Can you work these out from the model? Positions are in its coordinate system, mm. A direction names the side the tool comes from. Round coordinates to 2 decimals unless told otherwise and drop trailing zeros. Write each loop counter-clockwise with the first axis right and the second up, starting at its lowest first coordinate (ties: lowest second). Pieces come first, ordered by that corner, then holes. Notation, with made-up numbers: M 40.5,84.5 L 61.5,84.5 A4 ccw 61.5,90.5 Z; hole C 66.5,51.5 d9. An arc over 180 degrees is marked long. Answer as a JSON object with one key per item and string values. Group by question number.
1) If we mould it in two halves opening along Z, with no side actions, what happens to faces 4 (the flat face through (-35.2, 1, 13)), 5 (the flat face through (41.2, 1, -19)), 6 (the flat face through (39, 1, -12)), 7 (the flat face through (0, 1, 25))? For each: +Z half, -Z half, draft (parallel to the pull), parting line (faces both ways), or undercut.
2) Suppose I cut it at D-D, the plane y = 0.65. State how many separate pieces and enclosed holes the cut face has, and give its area (3 significant figures).
3) Suppose I cut it at B-B, the plane x = 30. Write out the boundary of the cut face in (y, z).
4) Suppose I cut it at A-A, the plane x = 19. Write out the boundary of the cut face in (y, z).
5) On a 3-axis mill with a long thin cutter (end or side, diameter ignored), from which of +Z, -Z, +X, -X, +Y, -Y can I reach the whole of each face in a straight line? I mean faces 1 (the flat face through (-40.2, 1, -19)), 2 (the flat face through (36.2, 1, -13)), 3 (the flat face through (31.2, 1, 16)). Say none if no direction works.
6) Suppose I cut it at C-C, the plane z = 0.05. Write out the boundary of the cut face in (x, y).
7) I'm going to push a flat-ended pin straight in: pin 1 Ø1 at (y, z) = (0.5, -13) entering from -X. Where does the tip first touch, or does it pass through?
8) Please list where these lines run through material, in increasing order: L1, parallel to Z at x = 30, y = 0.5; L2, parallel to X at y = 0.6, z = -17.5; L3, parallel to X at y = 0.65, z = -13.5. Write a range as [from, to].
from build123d import *

# Parameters (mm, degrees)
SKETCH2_W           = 100
SKETCH2_H           = 50
BOSS_EXTRUDE1_DEPTH = 2
SKETCH12_W          = 9.8
SKETCH12_H          = 50
SKETCH12_W_2        = 8.8
CUT_EXTRUDE8_DEPTH  = 6
SKETCH13_W          = 2
SKETCH13_H          = 7
SKETCH13_W_2        = 5
SKETCH13_H_2        = 2
CUT_EXTRUDE10_DEPTH = 6
SKETCH14_R          = 2
CUT_EXTRUDE11_DEPTH = 2


with BuildPart() as part:
    # Sketch2 → Boss-Extrude1 (new body)
    with BuildSketch(Plane(origin=(0, 0, 0), x_dir=(1, 0, 0), z_dir=(0, 1, 0))):
        Rectangle(SKETCH2_W, SKETCH2_H)
    extrude(amount=BOSS_EXTRUDE1_DEPTH)

    # Sketch12 → Cut-Extrude8 (cut)
    with BuildSketch(Plane(origin=(0, 2, 0), x_dir=(1, 0, 0), z_dir=(0, 1, 0))):
        with Locations((-45.1, 0)):
            Rectangle(SKETCH12_W, SKETCH12_H)
        with Locations((45.6, 0)):
            Rectangle(SKETCH12_W_2, SKETCH12_H)
    extrude(amount=-CUT_EXTRUDE8_DEPTH, mode=Mode.SUBTRACT)

    # Sketch13 → Cut-Extrude10 (cut)
    with BuildSketch(Plane(origin=(0, 2, 0), x_dir=(1, 0, 0), z_dir=(0, 1, 0))):
        with Locations((-29.2, 15.5)):
            Rectangle(SKETCH13_W, SKETCH13_H)
        with Locations((-29.2, 0)):
            Rectangle(SKETCH13_W, SKETCH13_H)
        with Locations((-29.2, -15.5)):
            Rectangle(SKETCH13_W, SKETCH13_H)
        with Locations((30.2, 15.5)):
            Rectangle(SKETCH13_W, SKETCH13_H)
        with Locations((30.2, 0)):
            Rectangle(SKETCH13_W, SKETCH13_H)
        with Locations((30.2, -15.5)):
            Rectangle(SKETCH13_W, SKETCH13_H)
        with Locations((-37.7, 13)):
            Rectangle(SKETCH13_W_2, SKETCH13_H_2)
        with Locations((-37.7, -13)):
            Rectangle(SKETCH13_W_2, SKETCH13_H_2)
        with Locations((38.7, 13)):
            Rectangle(SKETCH13_W_2, SKETCH13_H_2)
        with Locations((38.7, -13)):
            Rectangle(SKETCH13_W_2, SKETCH13_H_2)
    extrude(amount=-CUT_EXTRUDE10_DEPTH, mode=Mode.SUBTRACT)

    # Sketch14 → Cut-Extrude11 (cut)
    with BuildSketch(Plane.XZ):
        Polygon((25.004318917, -5.7), (20.125716489, -5.7), (20.125716489, -7.7), (27.496267271, -7.7), (24.06, 7.8), (10.849660593, 7.8), (7.413393322, -7.7), (14.783944105, -7.7), (14.783944105, -5.7), (9.905341676, -5.7), (12.454830297, 5.8), (22.454830297, 5.8), align=None)
        Polygon((14.783944105, -5.7), (20.125716489, -5.7), (25.004318917, -5.7), (22.454830297, 5.8), (12.454830297, 5.8), (9.905341676, -5.7), align=None)
        with Locations(Location((0.046267271, 0.05, 0), (0, 0, 270))):
            Circle(SKETCH14_R)
        with Locations(Location((38.046267271, 0.05, 0), (0, 0, 270))):
            Circle(SKETCH14_R)
    extrude(amount=-CUT_EXTRUDE11_DEPTH, mode=Mode.SUBTRACT)


solid = part.part
Results:
{
 "1": {"face 4": "undercut", "face 5": "draft", "face 6": "undercut", "face 7": "+Z half"},
 "2": {"separate pieces": "1", "enclosed holes": "9", "area": "3,670 mm^2"},
 "3": {"outline": "M 0,-25 L 2,-25 L 2,-19 L 0,-19 Z; M 0,-12 L 2,-12 L 2,-3.5 L 0,-3.5 Z; M 0,3.5 L 2,3.5 L 2,12 L 0,12 Z; M 0,19 L 2,19 L 2,25 L 0,25 Z"},
 "4": {"outline": "M 0,-25 L 2,-25 L 2,-5.7 L 0,-5.7 Z; M 0,7.8 L 2,7.8 L 2,25 L 0,25 Z"},
 "5": {"face 1": "+Z, -Z, -X, +Y, -Y", "face 2": "+X, +Y, -Y", "face 3": "+Y, -Y"},
 "6": {"outline": "M -40.2,0 L -30.2,0 L -30.2,2 L -40.2,2 Z; M -28.2,0 L -1.95,0 L -1.95,2 L -28.2,2 Z; M 2.05,0 L 9.13,0 L 9.13,2 L 2.05,2 Z; M 25.78,0 L 29.2,0 L 29.2,2 L 25.78,2 Z; M 31.2,0 L 36.05,0 L 36.05,2 L 31.2,2 Z; M 40.05,0 L 41.2,0 L 41.2,2 L 40.05,2 Z"},
 "7": {"pin 1": "x = -35.2"},
 "8": {"L1": "[-25, -19], [-12, -3.5], [3.5, 12], [19, 25]", "L2": "[-40.2, -30.2], [-28.2, 29.2], [31.2, 41.2]", "L3": "[-35.2, -30.2], [-28.2, 29.2], [31.2, 36.2]"}
}
